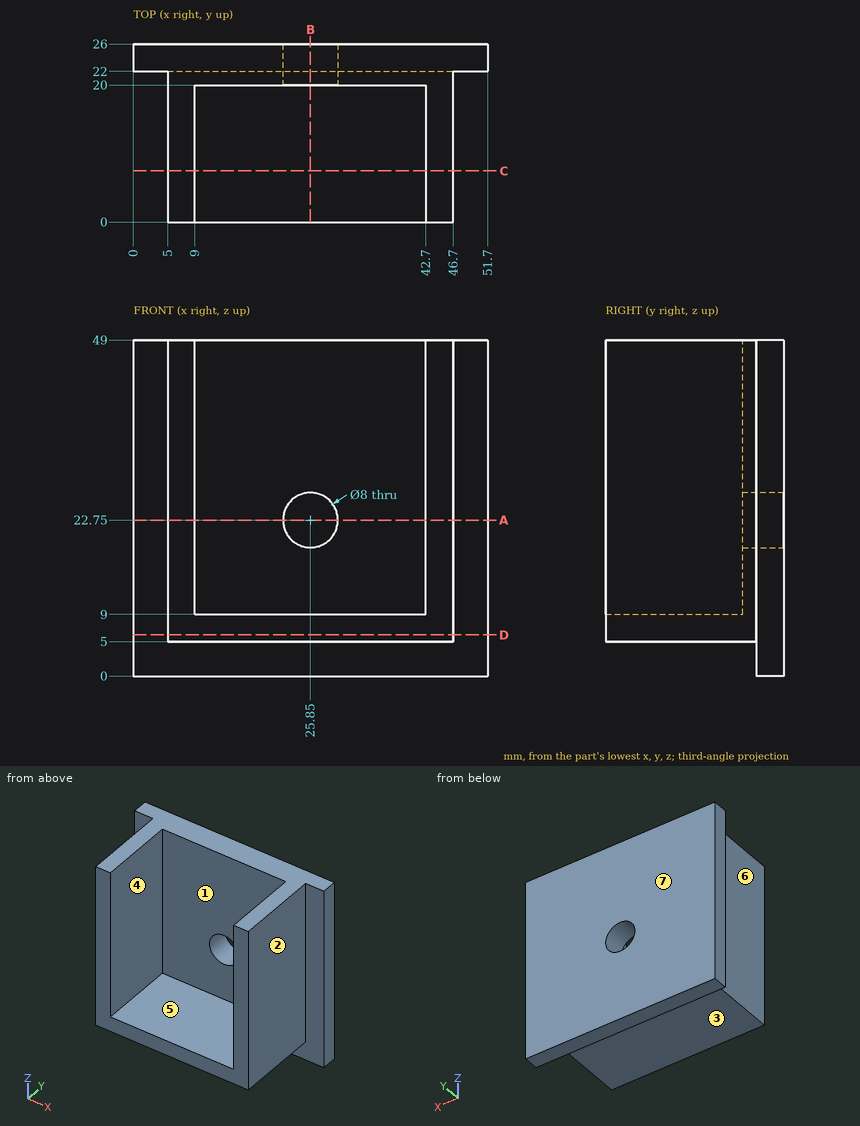
For this review, use the dimensioned drawing (mm, ordinates from the lowest corner) and the shaded views. A direction names the side the tool comes from. Round coordinates to 2 decimals unless told otherwise and drop trailing zeros. Write each loop counter-clockwise with the first axis right and the second up, starting at its lowest first coordinate (ties: lowest second). Pieces come first, ordered by that corner, then holes. Notation, with made-up numbers: (3, 20.5) -> (59, 20.5) arc R9 cw to (59, 27.5) -> close; hole circle Ø7 at (4, 72). An arc over 180 degrees is marked (long way). One line per item, written item: value. Start each with the question number.
Q1. To check wall thickness, follow probe 1 along X at (y, z) = (24.35, 22.75); probe 2 along X at (y, z) = (14, 12.5); probe 3 along Z at (x, y) = (17, 7.75). State the ranges of each line that lie inside material, in increasing order.
Q2. Add section B-B (x = 25.85). Give the boundary of the cut face in (y, z), then the cut area to 3 significant figures.
Q3. Add section A-A (z = 22.75). Give the boundary of the cut face in (x, y).
Q4. Add section C-C (y = 7.5). Give the boundary of the cut face in (x, z).
Q5. Add section D-D (z = 6). Give the boundary of the cut face in (x, y), then the cut area to 3 significant figures.
Q6. Tool access review of the marked faces 1, 2 and 3: name each direction out of +Z, -Z, +X, -X, +Y, -Y from which nothing blocks a thin tool from reaching the whole face with its end or side.
Q7. Insertion check: P1, Ø6.5, axis at x = 17, y = 9, coming from the -Z side; P2, Ø4, axis at y = 5.5, z = 7.5, coming from the +X side; P3, Ø2, axis at y = 23, z = 36.5, coming from the -X side; P4, Ø9, axis at x = 25.85, z = 22.75, coming from the -Y side. Each pin has a flat end and moves straight along its axis. Give the tip position at first contact, or say it passes through.
Q8. The part is to be moulded in two halves that separate along X. For the marked faces 4, 5, 6 and 7, say which applies: pulls with the +X half, pulls with the -X half, needs draft (parallel to the pull), parting line crosses it, or undercut.
Response:
1. probe 1: x = 0 to 21.85, 29.85 to 51.7
1. probe 2: x = 5 to 9, 42.7 to 46.7
1. probe 3: z = 5 to 9
2. outline: (0, 5) -> (22, 5) -> (22, 0) -> (26, 0) -> (26, 18.75) -> (20, 18.75) -> (20, 9) -> (0, 9) -> close; (20, 26.75) -> (26, 26.75) -> (26, 49) -> (20, 49) -> close
2. area: 316 mm^2
3. outline: (0, 22) -> (5, 22) -> (5, 0) -> (9, 0) -> (9, 20) -> (21.85, 20) -> (21.85, 26) -> (0, 26) -> close; (29.85, 20) -> (42.7, 20) -> (42.7, 0) -> (46.7, 0) -> (46.7, 22) -> (51.7, 22) -> (51.7, 26) -> (29.85, 26) -> close
4. outline: (5, 5) -> (46.7, 5) -> (46.7, 49) -> (42.7, 49) -> (42.7, 9) -> (9, 9) -> (9, 49) -> (5, 49) -> close
5. outline: (0, 22) -> (5, 22) -> (5, 0) -> (46.7, 0) -> (46.7, 22) -> (51.7, 22) -> (51.7, 26) -> (0, 26) -> close
5. area: 1,120 mm^2
6. face 1: +Z, -Y
6. face 2: +Z, -Z, +X, -Y
6. face 3: -Z, +X, -X, -Y
7. P1: stops at z = 5
7. P2: stops at x = 46.7
7. P3: stops at x = 0
7. P4: stops at y = 20
8. face 4: undercut
8. face 5: undercut
8. face 6: pulls with the -X half
8. face 7: needs draft
